Autodesk Inventor part; units mm, degrees
ref_plane "YZ Plane" through (0, 0, 0) normal (1, 0, 0) x (0, 1, 0)
ref_plane "XZ Plane" through (0, 0, 0) normal (0, 1, 0) x (-1, 0, 0)
ref_plane "XY Plane" through (0, 0, 0) normal (0, 0, 1) x (1, 0, 0)
sketch "Sketch4" plane through (0, 0, 0) normal (0, 0, 1) x (1, 0, 0)
  line L0 (-2.4, 0) -> (8, 0)
  line L1 (0, 0) -> (-2.4, 0)
  line L2 (0, 2.8) -> (0, 1.97)
  line L3 (0.5, 1.47) -> (0.5, 1.47)
  line L4 (0.5, 1.47) -> (1, 1.5)
  arc A0 (0, 1.97) -> (0.5, 1.47) centre (0.5, 1.97) ccw
  line L5 (-2.4, 0) -> (-2.4, 1.5)
  line L6 (0, 2.8) -> (-1.4761, 2.8)
  arc A1 (-1.4761, 2.8) -> (-2.4, 1.5) centre (2.0854, -0.7093) ccw
  line L7 (1, 1.5) -> (8, 1.5)
  line L8 (8, 1.5) -> (8, 0)
  point P0 (0, 1.47)
  dimension "d71" = 0.5
  dimension "d72" = 8
  dimension "d74" = 0.5
  dimension "d75" = 2.94
  dimension "d78" = 3
  dimension "d82" = 5
  dimension "d83" = 2.4
  dimension "d84" = 5.6
  dimension "d104" = 7
  dimension "d105" = 3
revolve "Revolution7" add sketch "Sketch4" angle 360 about axis through (-2.4, 0, 0) along (1, 0, 0)
sketch "Sketch5" plane through (-2.4, 0, 0) normal (-1, 0, 0) x (0, 0, 1)
  circle A0 centre (0, 0) radius 1.4 construction
  circle A1 centre (0, 0) radius 0.98 construction
  line L0 (0, 0) -> (-0.8487, 0.49)
  line L1 (0, 0) -> (-0.8487, -0.49)
  line L2 (-1.8008, 0) -> (1.7887, 0)
  line L3 (-1.4, 0) -> (-0.8487, -0.49)
  line L4 (-1.4, 0) -> (-0.8487, 0.49)
  point P0 (0, 0)
  dimension "d88" = 2.8
  dimension "d89" = 1.96
  dimension "d90" = 30
  dimension "d91" = 30
extrude "Extrusion1" cut sketch "Sketch5" against normal blind 1.27
pattern_circular "Circular Pattern1" count 6 over 360 about axis through (-10, 0, 0) along (1, 0, 0) of "Extrusion1"
fillet "Fillet1" radius 0.28 12 edges at (-1.765, -1.2124, -0.7) (-1.765, -0.49, -0.8487) (-1.765, -0.98, 0) (-1.765, -1.2124, 0.7) (-1.765, -0.49, 0.8487) (-1.765, 0, 1.4) (-1.765, 0.98, 0) (-1.765, 1.2124, 0.7) (-1.765, 0.49, 0.8487) (-1.765, 0.49, -0.8487) (-1.765, 0, -1.4) (-1.765, 1.2124, -0.7)
thread "Thread7"
properties part number "Šroub s válcovou hlavou a šestiramennou drážkou ISO 14583 - M3 x 8 - 4.8" material "Ocel"
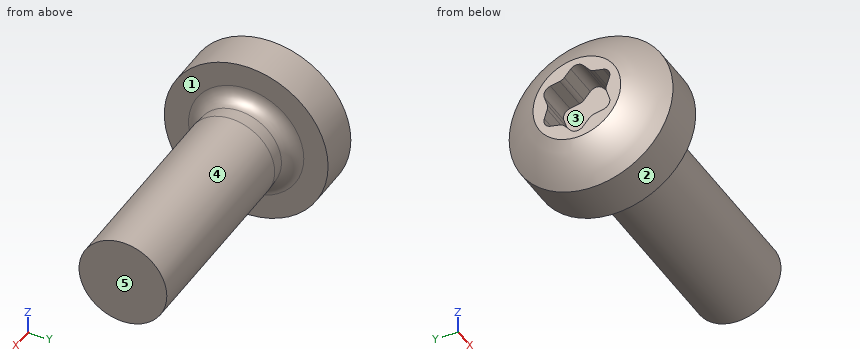
Can you work these out from the model? Positions are in its coordinate system, mm. Face numbers are marked on the shaded views. A direction names the side the tool comes from. Give positions to 0.01 mm unless a question says otherwise; leave off trailing zeros. Loops run counter-clockwise (first coordinate to the right, second up) from the corner with the lowest first, then second, coordinate; pieces in that order, holes last. Notation, with made-up numbers: (-4.75, 85) - (40.25, 85) arc R11 cw to (40.25, 90) - close; hole circle Ø1 at (40, 71.5). An arc over 180 degrees is marked (long way). Return JSON: item names as keys, results as strings.
1. I want a section at A-A on x = 1.5. Please give me the cut outline in (y, z).
Output values:
{"outline": "circle Ø3 at (0, 0)"}
2. If I drill on line 1 (Z direction, x = 2.5, y = -0.1); line 2 (X direction, y = -0.15, z = -0.05); line 3 (Y direction, x = -1.25, z = -1.1), over which ranges is the centre line in solid material (lowest first)?
Output values:
{"line 1": "z = -1.5 to 1.5", "line 2": "x = -1.13 to 8", "line 3": "y = -2.57 to -0.27, 0.27 to 2.57"}
3. For the marked faces 4 and 5, which set-ups out of +Z, -Z, +X, -X, +Y, -Y let a thin tool reach every point of the face, with its end or its side?
Output values:
{"face 4": "+X", "face 5": "+Z, -Z, +X, +Y, -Y"}
4. We'd pull the mould along Z, two halves only. Please class the marked faces 1, 2 and 3: +Z half, -Z half, draft (parallel to the pull), parting line (faces both ways), or undercut.
Output values:
{"face 1": "draft", "face 2": "parting line", "face 3": "undercut"}
5. I'm going to push a flat-ended pin straight in: pin 1 Ø1 at (x, y) = (0, -0.5) entering from -Z. Where does the tip first touch, or does it pass through?
Output values:
{"pin 1": "stops at z = -2.8"}
